from build123d import *

# Parameters (mm, degrees)
SKETCH1_W               = 22.2
SKETCH1_H               = 9
SKETCH1_R               = 1.5
BOSS_EXTRUDE1_DEPTH     = 3
SKETCH2_W               = 3
SKETCH2_H               = 9
BOSS_EXTRUDE2_DEPTH     = 3
BOSS_EXTRUDE3_START     = -10.35
BOSS_EXTRUDE3_OUTLINE_R = 0.75
BOSS_EXTRUDE3_DEPTH     = 1.5
SKETCH4_W               = 8.1
SKETCH4_H               = 9
BOSS_EXTRUDE4_DEPTH     = 7.35
CHAMFER1_SIZE           = 7.35
CHAMFER2_SIZE           = 4.5
CUT_EXTRUDE1_START      = -3
SKETCH5_R               = 3
CUT_EXTRUDE1_DEPTH      = 16.180349282


# Read off the part's stored shape, not the designer's step: Boss-Extrude3
with BuildPart() as part:
    # Sketch1 → Boss-Extrude1 (new body)
    with BuildSketch(Plane(origin=(0, 0, 0), x_dir=(1, 0, 0), z_dir=(0, 1, 0))):
        Rectangle(SKETCH1_W, SKETCH1_H)
        with Locations(Location((0, 0, 0), (0, 0, 270))):
            Circle(SKETCH1_R, mode=Mode.SUBTRACT)
    extrude(amount=BOSS_EXTRUDE1_DEPTH)

    # Sketch2 → Boss-Extrude2 (add)
    with BuildSketch(Plane(origin=(0, 3, 0), x_dir=(1, 0, 0), z_dir=(0, 1, 0))):
        with Locations((-9.6, 0)):
            Rectangle(SKETCH2_W, SKETCH2_H)
        with Locations((9.6, 0)):
            Rectangle(SKETCH2_W, SKETCH2_H)
    extrude(amount=BOSS_EXTRUDE2_DEPTH)



with BuildPart() as body_2:
    # Boss-Extrude3 outline → Boss-Extrude3 (new body)
    with BuildSketch(Plane(origin=(0, 3, 0), x_dir=(1, 0, 0), z_dir=(0, 1, 0)).offset(BOSS_EXTRUDE3_START)):
        with BuildLine():
            Line((-12, -4.51), (-11.1, -4.5))
            Line((-11.1, -4.5), (-11.1, 0))
            Line((-11.1, 0), (-12, -0.01))
            ThreePointArc((-12, -0.01), (-14.25, -2.26), (-12, -4.51))
        make_face()
        with Locations((-12, -2.26)):
            Circle(BOSS_EXTRUDE3_OUTLINE_R, mode=Mode.SUBTRACT)
    extrude(amount=BOSS_EXTRUDE3_DEPTH)


with BuildPart() as part_1:
    add(part.part)

    add(body_2.part)  # Boss-Extrude4 merges body 2
    # Sketch4 → Boss-Extrude4 (add)
    with BuildSketch(Plane.XZ):
        with Locations((-7.05, 0)):
            Rectangle(SKETCH4_W, SKETCH4_H)
    extrude(amount=BOSS_EXTRUDE4_DEPTH)

    # Chamfer1
    # the kernel refuses this chamfer: 7.35 mm, written as the material it adds along each edge
    with BuildSketch(Plane(origin=(-3, 0, 4.5), x_dir=(0.9996219169112966, 0.027495876610586372, 0), z_dir=(0, 0, -1))) as chamfer1_piece_1_section:
        Polygon((CHAMFER1_SIZE * 0.999621916911, CHAMFER1_SIZE * 0.0274958766106), (-CHAMFER1_SIZE * 0.0274958766106, CHAMFER1_SIZE * 0.999621916911), (0, 0), align=None)
    chamfer1_piece_1 = extrude(amount=9, mode=Mode.PRIVATE)
    chamfer1_piece_1 = chamfer1_piece_1 - Plane(origin=(0, -1.008100378, 0), x_dir=(0, 0, 1), z_dir=(0, -1, 0)) * Cylinder(1.5, 48, mode=Mode.PRIVATE)
    chamfer1_piece_1 = split(chamfer1_piece_1, bisect_by=Plane(origin=(3.254582701, -7.35, -3), z_dir=(0, 1, 0)), keep=Keep.TOP, mode=Mode.PRIVATE)
    add(chamfer1_piece_1)

    # Chamfer2
    chamfer2_edges = [part_1.edges().sort_by_distance(p)[0] for p in [
        (-7.05, -7.35, -4.5),
    ]]
    chamfer(chamfer2_edges, length=CHAMFER2_SIZE)

    # Sketch5 → Cut-Extrude1 (cut, through all)
    with BuildSketch(Plane(origin=(0, 3, 0), x_dir=(1, 0, 0), z_dir=(0, 1, 0)).offset(CUT_EXTRUDE1_START)):
        with Locations(Location((0, 0, 0), (0, 0, 270))):
            Circle(SKETCH5_R)
    extrude(amount=-CUT_EXTRUDE1_DEPTH, mode=Mode.SUBTRACT)


solid = part_1.part
Could you check a few things on this model? Use its own coordinates, in mm. A direction names the side the tool comes from. Give positions to 0.01 mm unless a question says otherwise; leave off trailing zeros. Write each loop counter-clockwise with the first axis right and the second up, starting at its lowest first coordinate (ties: lowest second). Pieces come first, ordered by that corner, then holes. Notation, with made-up numbers: (2.25, 3) -> (57.25, 3) arc R28 cw to (57.25, 42) -> close; hole circle Ø2 at (-17.5, 32.25). An arc over 180 degrees is marked (long way). Write each question's results on one line, items separated by ' | '. Start each with the question number.
Q1. Suppose I cut it at D-D, the plane z = -3.25. List the corners of the cut face in (x, y) for me, and give its area (3 significant figures).
Q2. We'd pull the mould along Z, two halves only. Please class faces 1 (the face through (-2.93, -2.81, -0.65)), 2 (the face through (-3, -1, 4.5)), 3 (the face through (0.45, 1.48, 1.43)), 4 (the face through (10, 6, 0)): +Z half, -Z half, draft (parallel to the pull), parting line (faces both ways), or undercut.
Q3. Suppose I cut it at B-B, the plane z = -1. List the corners of the cut face in (x, y) for me, and give its area (3 significant figures).
Q4. I'm going to push flat-ended pins straight in: pin 1 Ø3 at (y, z) = (1.5, -1) entering from -X; pin 2 Ø1 at (x, y) = (0, -4) entering from -Z; pin 3 Ø1.4 at (x, z) = (-12, 2.26) entering from -Y; pin 4 Ø4 at (x, z) = (4.5, -1.5) entering from +Y. Where does each tip first touch, or does it pass through?
Q5. I need wall thicknesses on probe 1 along X at (y, z) = (4.5, 3.5); probe 2 along Z at (x, y) = (-12, -6.6); probe 3 along X at (y, z) = (1.7, 0). Which ranges of each line are inside material? Lowest first, please.
Q6. Which directions (+Z, -Z, +X, -X, +Y, -Y) give clear straight access to the entire face, cutting with the end or side of a thin tool? Please do faces 5 (the face through (8, 0, 0)), 6 (the face through (-1.3, 0, 1.3)), 7 (the face through (-8.1, 4, 0)).
Q7. Suppose I cut it at A-A, the plane y = 3.5. List the corners of the cut face in (x, z) for me, and give its area (3 significant figures).
Q8. Suppose I cut it at C-C, the plane x = -12.5. List the corners of the cut face in (y, z) for me.
Outcome:
1) outline: (-11.1, -4.1) -> (0.25, -4.1) -> (4.35, 0) -> (11.1, 0) -> (11.1, 6) -> (8.1, 6) -> (8.1, 3) -> (-8.1, 3) -> (-8.1, 6) -> (-11.1, 6) -> close | area: 140 mm2
2) face 1: undercut | face 2: +Z half | face 3: undercut | face 4: draft
3) outline: (-11.1, -6.35) -> (-2.83, -6.35) -> (-2.83, 0) -> (-1.12, 0) -> (-1.12, 3) -> (-8.1, 3) -> (-8.1, 6) -> (-11.1, 6) -> close; (1.12, 0) -> (2.83, 0) -> (2.83, -1.52) -> (4.35, 0) -> (11.1, 0) -> (11.1, 6) -> (8.1, 6) -> (8.1, 3) -> (1.12, 3) -> close | area: 132 mm2
4) pin 1: x = -11.1 | pin 2: z = -3.85 | pin 3: through | pin 4: y = 3
5) probe 1: -11.1 to -8.1, 8.1 to 11.1 | probe 2: 0.01 to 1.51, 3.01 to 4.51 | probe 3: -11.1 to -1.5, 1.5 to 11.1
6) face 5: +Z, -Z, +X, -Y | face 6: -Y | face 7: +Z, -Z, +Y
7) outline: (-11.1, -4.5) -> (-8.1, -4.5) -> (-8.1, 4.5) -> (-11.1, 4.5) -> close; (8.1, -4.5) -> (11.1, -4.5) -> (11.1, 4.5) -> (8.1, 4.5) -> close | area: 54.0 mm2
8) outline: (-7.35, 0.07) -> (-5.85, 0.07) -> (-5.85, 1.7) -> (-7.35, 1.7) -> close; (-7.35, 2.82) -> (-5.85, 2.82) -> (-5.85, 4.45) -> (-7.35, 4.45) -> close
